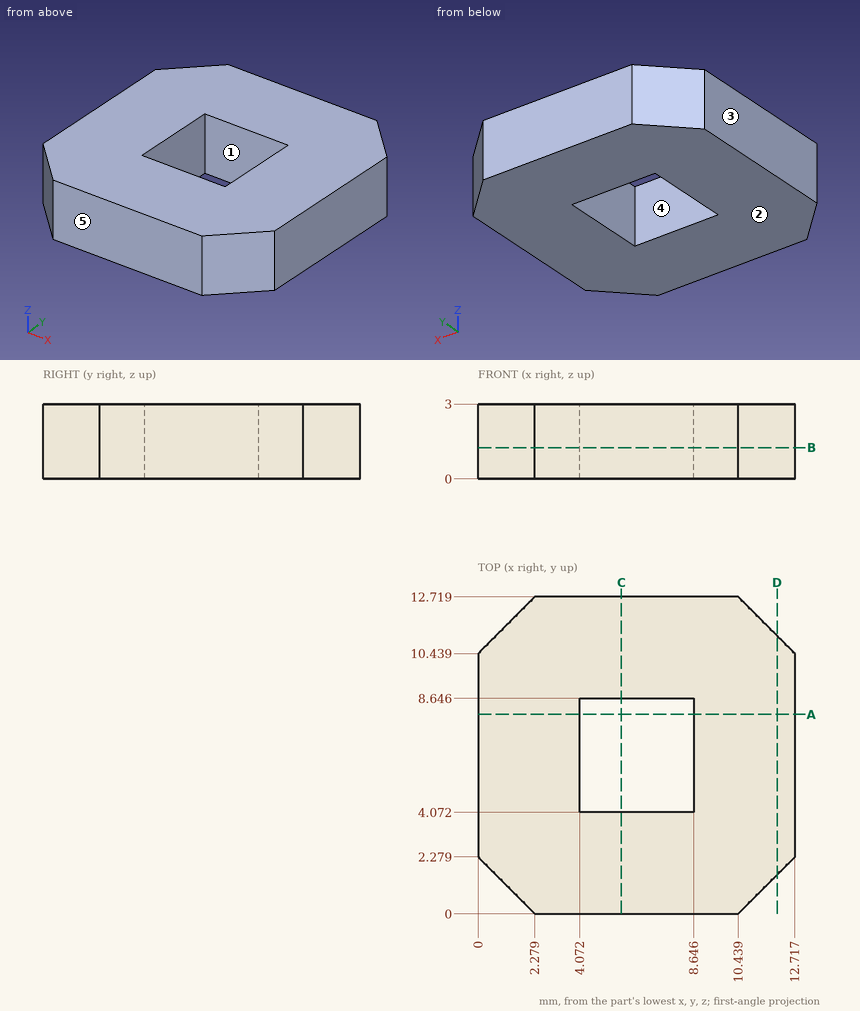
Study the drawing (mm; zero at the part's minimum x, y, z) and answer. A direction names the side the tool comes from. Give positions to 0.01 mm unless a question says otherwise; leave off trailing zeros. Loops run counter-clockwise (first coordinate to the right, second up) from the corner with the lowest first, then second, coordinate; pieces in that order, holes last. Notation, with made-up numbers: (-37.75, 35.25) - (6.25, 35.25) arc R10 cw to (6.25, 49.25) - close; hole circle Ø7 at (1.25, 33.25). An arc over 180 degrees is marked (long way). Answer in a Markdown table with one row per item. Add a question column.
Q1. Determine the mould class of the marked faces 3, 4 and 5 for opening direction X: released by +X, released by -X, zero draft, split by the parting line, or undercut.
Q2. The part is cut by section C-C (x = 5.75). Determine the outline of the cut face in (y, z).
Q3. The part is cut by section A-A (y = 8). Determine the outline of the cut face in (x, z) (1 decimal).
Q4. Consider line 1 along X through (y, z) = (7.5, 2.1) (1 decimal); line 2 along Y through (x, z) = (6.75, 0.3); line 3 along X through (y, z) = (11.5, 0.65) (1 decimal). Determine where each line is inside the solid, lowest interval first.
Q5. A tool of negligible diameter and unlimited length cuts with its end or side. For the marked faces 1 and 2, from which of +Z, -Z, +X, -X, +Y, -Y can it reach the whole face along a straight path? Write none if from no direction.
Q6. The part is cut by section B-B (z = 1.25). Determine the outline of the cut face in (x, y) (1 decimal), and give its area (3 significant figures).
Q7. The part is cut by section D-D (x = 12). Determine the outline of the cut face in (y, z), and give its area (3 significant figures).
Solution:
| question | item | result |
|---|---|---|
| 1 | face 3 | released by -X |
| 1 | face 4 | undercut |
| 1 | face 5 | zero draft |
| 2 | outline | (0, 0) - (4.07, 0) - (4.07, 3) - (0, 3) - close; (8.65, 0) - (12.72, 0) - (12.72, 3) - (8.65, 3) - close |
| 3 | outline | (0, 0) - (4.1, 0) - (4.1, 3) - (0, 3) - close; (8.6, 0) - (12.7, 0) - (12.7, 3) - (8.6, 3) - close |
| 4 | line 1 | x = 0 to 4.1, 8.6 to 12.7 |
| 4 | line 2 | y = 0 to 4.07, 8.65 to 12.72 |
| 4 | line 3 | x = 1.1 to 11.7 |
| 5 | face 1 | +Z, -Z |
| 5 | face 2 | -Z, +X, -X, +Y, -Y |
| 6 | outline | (0, 2.3) - (2.3, 0) - (10.4, 0) - (12.7, 2.3) - (12.7, 10.4) - (10.4, 12.7) - (2.3, 12.7) - (0, 10.4) - close; hole (4.1, 4.1) - (8.6, 4.1) - (8.6, 8.6) - (4.1, 8.6) - close |
| 6 | area | 130 mm² |
| 7 | outline | (1.56, 0) - (11.16, 0) - (11.16, 3) - (1.56, 3) - close |
| 7 | area | 28.8 mm² |
